Autodesk Inventor part; units mm, degrees
ref_plane "YZ Plane" through (0, 0, 0) normal (1, 0, 0) x (0, 1, 0)
ref_plane "XZ Plane" through (0, 0, 0) normal (0, 1, 0) x (-1, 0, 0)
ref_plane "XY Plane" through (0, 0, 0) normal (0, 0, 1) x (1, 0, 0)
sketch "Boceto1" plane through (0, 0, 0) normal (0, 1, 0) x (-1, 0, 0)
  circle A0 centre (0, 0) radius 20
  dimension "d0" = 40
extrude "Extrusión1" add sketch "Boceto1" along normal blind 60
sketch "Boceto10" plane through (0, 0, 0) normal (0, -1, 0) x (1, 0, 0)
  circle A0 centre (0, 0) radius 11
  dimension "d34" = 22
extrude "Extrusión2" cut sketch "Boceto10" against normal blind 35
sketch "Boceto11" plane through (0, 0, 0) normal (1, 0, 0) x (0, 1, 0)
  line L0 (35, -11) -> (35, 11)
  line L1 (35, 0) -> (35, 11)
  line L2 (35, 0) -> (45, 0)
  line L3 (45, 0) -> (45, 5)
  line L4 (45, 5) -> (35, 11)
  point P0 (0, 0)
  dimension "d37" = 10
  dimension "d38" = 5
revolve "Revolución6" cut sketch "Boceto11" angle 360 about axis through (0, 35, 0) along (0, -1, 0)
sketch "Boceto12" plane through (0, 45, 0) normal (0, -1, 0) x (1, 0, 0)
  circle A0 centre (0, 0) radius 5
extrude "Extrusión3" cut sketch "Boceto12" against normal blind 35
sketch "Boceto13" plane through (0, 60, 0) normal (0, 1, 0) x (1, 0, 0)
  circle A0 centre (0, 0) radius 5
  circle A1 centre (0, 0) radius 20
  dimension "d42" = 40
extrude "Extrusión4" cut sketch "Boceto13" against normal blind 1
sketch "Boceto14" plane through (0, 60, 0) normal (0, 1, 0) x (1, 0, 0)
  circle A0 centre (0, 0) radius 27.5
  dimension "d45" = 55
extrude "Extrusión5" add sketch "Boceto14" against normal blind 3
sketch "Boceto15" plane through (0, 57, 0) normal (0, -1, 0) x (1, 0, 0)
  circle A0 centre (0, 0) radius 11
  circle A1 centre (0, 0) radius 5
extrude "Extrusión6" cut sketch "Boceto15" against normal blind 10 contours A1
sketch "Boceto16" plane through (0, 0, 0) normal (0, -1, 0) x (1, 0, 0)
  circle A0 centre (0, 0) radius 27.5
  circle A1 centre (0, 0) radius 17.05
  dimension "d50" = 34.1
extrude "Extrusión7" add sketch "Boceto16" along normal blind 3
sketch "Boceto17" plane through (0, 60, 0) normal (0, 1, 0) x (1, 0, 0)
  circle A0 centre (0, 0) radius 20
  circle A1 centre (0, 0) radius 27.5
  circle A2 centre (0, -23.75) radius 2.75
  circle A3 centre (-23.75, 0) radius 2.75
  circle A4 centre (0, 23.75) radius 2.75
  circle A5 centre (23.75, 0) radius 2.75
  dimension "d53" = 40
  dimension "d58" = 5.5
  dimension "d59" = 5.5
  dimension "d60" = 5.5
  dimension "d61" = 5.5
extrude "Extrusión8" cut sketch "Boceto17" against normal blind 100 contours A2 | A3 | A4 | A5
sketch "Boceto18" plane through (0, 60, 0) normal (0, 1, 0) x (1, 0, 0)
  circle A0 centre (0, 0) radius 11.5
  dimension "d64" = 23
extrude "Extrusión9" cut sketch "Boceto18" against normal blind 7
properties part number "cabezal extrusora"
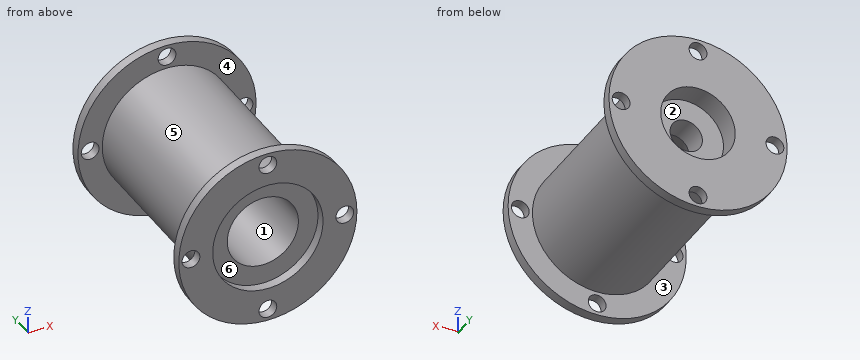
CAD build for the part. Positions are in the model's coordinates, mm. Face numbers are marked on the shaded views. A direction names the side the tool comes from. Coordinates: 2 decimals unless noted, no trailing zeros. Loops run counter-clockwise (first coordinate to the right, second up) from the corner with the lowest first, then second, coordinate; pieces in that order, holes last. Notation, with made-up numbers: (55, 3) - (87, 3) arc R25 ccw to (87, 39) - close; hole circle Ø9 at (-10, -23.75). An arc over 180 degrees is marked (long way). Use CSV: the item, a comma, the result in double quotes. Start each with the question number.
Q1. Cut at B-B, the plane y = 25.5. List the corners of the cut face in (x, z), then the cut area to 3 significant figures.
Q2. Drop flat-ended pins along their axis: P1, Ø1.5, axis at y = 8.5, z = -10.5, coming from the -X side; P2, Ø13, axis at x = 0, z = 0, coming from the +Y side; P3, Ø5, axis at y = 5.5, z = -2.5, coming from the -X side; P4, Ø3.5, axis at x = -23.75, z = 0, coming from the -Y side. Give the stop position or say it passes through.
Q3. Cut at D-D, the plane z = 0. State how many separate pieces and enclosed holes the cut face has, then the cut area to 3 significant figures.
Q4. 3-axis set-ups, long thin cutter, end or side, ignore diameter. For the marked faces 1, 2 and 3: which of +Z, -Z, +X, -X, +Y, -Y reach the whole face in a straight line?
Q5. Probe probe 1 along Z at (x, y) = (0, 59.2); probe 2 along Z at (x, y) = (0, -1); probe 3 along Y at (x, z) = (14.5, 22). List the from-to ranges inside material, lowest first. Write a range as from..to.
Q6. Cut at C-C, the plane x = 23.75. List the corners of the cut face in (y, z), then the cut area to 3 significant figures.
Q7. Two-plate mould, pull along Z, no slides. Class the marked faces 4, 5 and 6: +Z half, -Z half, draft (parallel to the pull), parting line (faces both ways), or undercut.
Q8. Cut at A-A, the plane z = 23.75. List the corners of the cut face in (x, y).
Here are the results:
1,outline,"circle Ø40 at (0, 0); hole circle Ø22 at (0, 0)"
1,area,"877 mm2"
2,P1,"x = -17.46"
2,P2,"y = 53"
2,P3,"x = -20"
2,P4,"through"
3,separate pieces,"6"
3,enclosed holes,"0"
3,area,"1,270 mm2"
4,face 1,"-Y"
4,face 2,"+Y"
4,face 3,"none"
5,probe 1,"-27.5..-26.5, -21..-11.5, 11.5..21, 26.5..27.5"
5,probe 2,"-27.5..-26.5, -21..-17.05, 17.05..21, 26.5..27.5"
5,probe 3,"-3..0, 57..60"
6,outline,"(-3, -13.86) - (0, -13.86) - (0, -2.75) - (-3, -2.75) - close; (-3, 2.75) - (0, 2.75) - (0, 13.86) - (-3, 13.86) - close; (57, -13.86) - (60, -13.86) - (60, -2.75) - (57, -2.75) - close; (57, 2.75) - (60, 2.75) - (60, 13.86) - (57, 13.86) - close"
6,area,"133 mm2"
7,face 4,"draft"
7,face 5,"parting line"
7,face 6,"undercut"
8,outline,"(-13.86, -3) - (-2.75, -3) - (-2.75, 0) - (-13.86, 0) - close; (-13.86, 57) - (-2.75, 57) - (-2.75, 60) - (-13.86, 60) - close; (2.75, -3) - (13.86, -3) - (13.86, 0) - (2.75, 0) - close; (2.75, 57) - (13.86, 57) - (13.86, 60) - (2.75, 60) - close"
